```python
from build123d import *

# Parameters (mm, degrees)
SKETCH034_W     = 35
SKETCH034_H     = 30
PAD022_DEPTH    = 4
SKETCH035_W     = 4.5
SKETCH035_H     = 28
POCKET009_DEPTH = 3
SKETCH036_W     = 3
SKETCH036_H     = 3
PAD023_DEPTH    = 0.5


with BuildPart() as part:
    # Sketch034 (on Face1 of CopyPad014001) → Pad022 (new body)
    with BuildSketch(Plane.XY.offset(1.2)):
        with Locations((19.5, 26.55)):
            Rectangle(SKETCH034_W, SKETCH034_H)
    extrude(amount=PAD022_DEPTH)

    # Sketch035 (on Face6 of Pad022) → Pocket009 (cut)
    with BuildSketch(Plane.XY.offset(5.2)):
        with Locations((34.75, 26.55)):
            Rectangle(SKETCH035_W, SKETCH035_H)
    extrude(amount=-POCKET009_DEPTH, mode=Mode.SUBTRACT)

    # Sketch036 (on Face8 of Pocket009) → Pad023 (join)
    with BuildSketch(Plane.XY.offset(2.2)):
        with Locations((34.75, 34.05)):
            Rectangle(SKETCH036_W, SKETCH036_H)
        with Locations((34.75, 19.05)):
            Rectangle(SKETCH036_W, SKETCH036_H)
    extrude(amount=PAD023_DEPTH)


solid = part.part
```
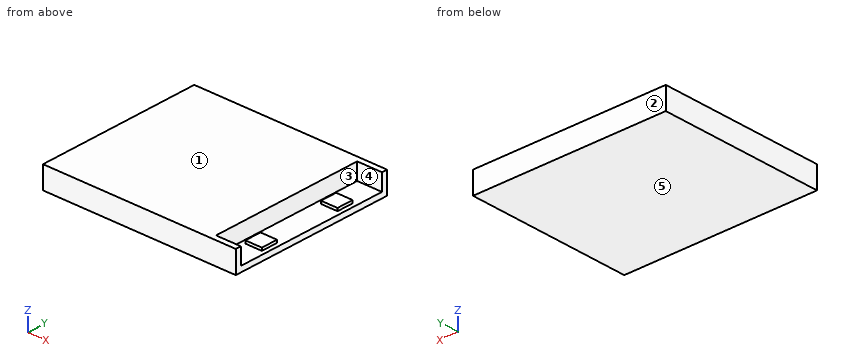
Here's how the part is built. I have some questions about the finished solid (model axes, mm). Face numbers are marked on the shaded views. A direction names the side the tool comes from. Give positions to 0.01 mm unless a question says otherwise; leave off trailing zeros. Write each loop counter-clockwise with the first axis right and the second up, starting at its lowest first coordinate (ties: lowest second). Pieces come first, ordered by that corner, then holes.
(1) Imagine slicing it at B-B, the plane z = 4.7. Write out the boundary of the cut face in (x, y), and give its area (3 significant figures).
Output values:
outline: (2, 11.55) - (37, 11.55) - (37, 12.55) - (32.5, 12.55) - (32.5, 40.55) - (37, 40.55) - (37, 41.55) - (2, 41.55) - close
area: 924 mm2
(2) Thinking about a two-plate mould opening in Y: for the marked faces 1, 2 and 3, which applies, pulls with the +Y half, pulls with the -Y half, needs draft (parallel to the pull), parting line crosses it, or undercut?
Output values:
face 1: needs draft
face 2: pulls with the +Y half
face 3: undercut
(3) On a 3-axis mill with a long thin cutter (end or side, diameter ignored), from which of +Z, -Z, +X, -X, +Y, -Y can I reach the whole of each face in a straight line? I mean the marked faces 4 and 5. Say none if no direction works.
Output values:
face 4: +Z, +X
face 5: -Z, +X, -X, +Y, -Y
(4) If I drill on L1, parallel to Y at x = 33.5, z = 2.25; L2, parallel to Z at x = 33, y = 25.5; L3, parallel to X at y = 36.75, z = 4.3, over which ranges is the centre line in solid material (lowest first)?
Output values:
L1: y = 11.55 to 12.55, 17.55 to 20.55, 32.55 to 35.55, 40.55 to 41.55
L2: z = 1.2 to 2.2
L3: x = 2 to 32.5
(5) Will this pin go through, and if not, where does the flat tip stop? pin 1 (3.5 mm diameter, centred on x = 34.5, y = 18.5, fed in from +Z).
Output values:
pin 1: stops at z = 2.7
(6) Imagine slicing it at A-A, the plane x = 35.5. Write out the boundary of the cut face in (y, z), and give its area (3 significant figures).
Output values:
outline: (11.55, 1.2) - (41.55, 1.2) - (41.55, 5.2) - (40.55, 5.2) - (40.55, 2.2) - (35.55, 2.2) - (35.55, 2.7) - (32.55, 2.7) - (32.55, 2.2) - (20.55, 2.2) - (20.55, 2.7) - (17.55, 2.7) - (17.55, 2.2) - (12.55, 2.2) - (12.55, 5.2) - (11.55, 5.2) - close
area: 39.0 mm2
(7) Imagine slicing it at C-C, the plane y = 21. Write out the boundary of the cut face in (x, z).
Output values:
outline: (2, 1.2) - (37, 1.2) - (37, 2.2) - (32.5, 2.2) - (32.5, 5.2) - (2, 5.2) - close
